Build history of the part. All positions in model axes, mm. Face numbers are marked on the shaded views. Round coordinates to 2 decimals unless told otherwise and drop trailing zeros. Order: outer loops, then holes, each group sorted by start corner. A loop starts at its lowest first (then second) coordinate and runs counter-clockwise, first axis right, second up. Notation, with made-up numbers: M 29,-13.5 L 45,-13.5 A25 cw 45,25.5 Z; hole C 69.25,75.25 d3. An arc over 180 degrees is marked long. One line per item, written item: value. Start each with the question number.
Item 1: Band-saw the part on A-A, the plane y = 20. Write the cut outline in (x, z), then the cut area to 3 significant figures.
Item 2: Probe L1, parallel to Y at x = -20, z = 1.15; L2, parallel to Y at x = 24, z = 8. List the from-to ranges inside material, lowest first.
Item 3: Band-saw the part on B-B, the plane x = 20. Write the cut outline in (y, z).
Item 4: Pin check, flat tips, straight feed: pin 1 (3.5 mm diameter, centred on x = 20, y = -20, fed in from +Z); pin 2 (8 mm diameter, centred on x = -20, y = 20, fed in from +Z). Stop position of each tip, or through.
Item 5: Band-saw the part on D-D, the plane y = 7. Write the cut outline in (x, z), then the cut area to 3 significant figures.
Item 6: Band-saw the part on C-C, the plane z = 3.25. Write the cut outline in (x, y), then the cut area to 3 significant figures.
Item 7: Two-plate mould, pull along X, no slides. Class the marked faces 1, 2, 3 and 4: +X half, -X half, draft (parallel to the pull), parting line (faces both ways), or undercut.
```python
from build123d import *

# Parameters (mm, degrees)
SKETCH_W        = 60
SKETCH_H        = 60
PAD_DEPTH       = 10
SKETCH001_W     = 55
SKETCH001_H     = 55
POCKET_DEPTH    = 5
FILLET_R        = 2
FILLET001_R     = 2
FILLET002_R     = 2
FILLET003_R     = 2
SKETCH002_R     = 3
HOLE_DEPTH      = 25
SKETCH003_W     = 10
SKETCH003_H     = 3
POCKET001_DEPTH = 5


with BuildPart() as part:
    # Sketch → Pad (new body)
    with BuildSketch(Plane.XY):
        Rectangle(SKETCH_W, SKETCH_H)
    extrude(amount=PAD_DEPTH)

    # Sketch001 (on Face6 of Pad) → Pocket (cut)
    with BuildSketch(Plane.XY.offset(10)):
        Rectangle(SKETCH001_W, SKETCH001_H)
    extrude(amount=-POCKET_DEPTH, mode=Mode.SUBTRACT)

    # Fillet
    fillet_edges = [part.edges().sort_by_distance(p)[0] for p in [
        (-27.5, 27.5, 7.5),
    ]]
    fillet(fillet_edges, radius=FILLET_R)

    # Fillet001
    fillet001_edges = [part.edges().sort_by_distance(p)[0] for p in [
        (27.5, 27.5, 7.5),
    ]]
    fillet(fillet001_edges, radius=FILLET001_R)

    # Fillet002
    fillet002_edges = [part.edges().sort_by_distance(p)[0] for p in [
        (-27.5, -27.5, 7.5),
    ]]
    fillet(fillet002_edges, radius=FILLET002_R)

    # Fillet003
    fillet003_edges = [part.edges().sort_by_distance(p)[0] for p in [
        (27.5, -27.5, 7.5),
    ]]
    fillet(fillet003_edges, radius=FILLET003_R)

    # Sketch002 (on Face14 of Fillet003) → Hole (cut)
    with BuildSketch(Plane.XY.offset(5)):
        with Locations((-20, 20)):
            Circle(SKETCH002_R)
        with Locations((-20, -20)):
            Circle(SKETCH002_R)
        with Locations((20, -20)):
            Circle(SKETCH002_R)
        with Locations((20, 20)):
            Circle(SKETCH002_R)
    extrude(amount=-HOLE_DEPTH, mode=Mode.SUBTRACT)

    # Sketch003 (on Face1 of Hole) → Pocket001 (cut)
    with BuildSketch(Plane.XY.offset(10)):
        with Locations((18, 28.5)):
            Rectangle(SKETCH003_W, SKETCH003_H)
    extrude(amount=-POCKET001_DEPTH, mode=Mode.SUBTRACT)


solid = part.part
```
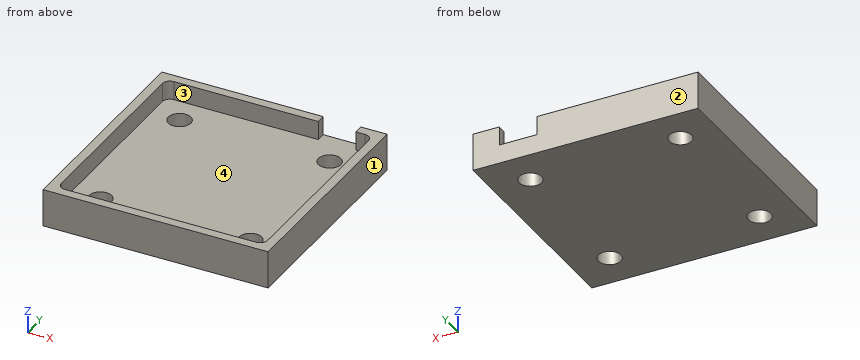
Output:
1. outline: M -30,0 L -23,0 L -23,5 L -27.5,5 L -27.5,10 L -30,10 Z; M -17,0 L 17,0 L 17,5 L -17,5 Z; M 23,0 L 30,0 L 30,10 L 27.5,10 L 27.5,5 L 23,5 Z
1. area: 265 mm²
2. L1: y = -30 to -23, -17 to 17, 23 to 30
2. L2: y = -30 to -27.5, 27.5 to 30
3. outline: M -30,0 L -23,0 L -23,5 L -27.5,5 L -27.5,10 L -30,10 Z; M -17,0 L 17,0 L 17,5 L -17,5 Z; M 23,0 L 30,0 L 30,5 L 23,5 Z
4. pin 1: passes through
4. pin 2: stops at z = 5
5. outline: M -30,0 L 30,0 L 30,10 L 27.5,10 L 27.5,5 L -27.5,5 L -27.5,10 L -30,10 Z
5. area: 325 mm²
6. outline: M -30,-30 L 30,-30 L 30,30 L -30,30 Z; hole C -20,-20 d6; hole C -20,20 d6; hole C 20,-20 d6; hole C 20,20 d6
6. area: 3,490 mm²
7. face 1: +X half
7. face 2: draft
7. face 3: undercut
7. face 4: undercut
